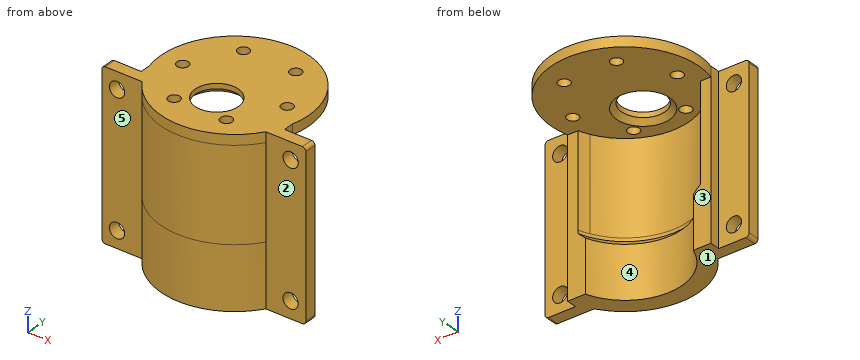
from build123d import *
from build123d.topology import SkipClean

# Parameters (mm, degrees)
BOSS_EXTRUDE1_START     = 94
SKETCH1_R               = 21.9
SKETCH1_R_2             = 1.7
SKETCH1_R_3             = 6.4
BOSS_EXTRUDE1_DEPTH     = 3
BOSS_EXTRUDE2_START     = 91
BOSS_EXTRUDE2_DEPTH     = 27.5
BOSS_EXTRUDE3_START     = 45
BOSS_EXTRUDE3_DEPTH     = 18.5
BOSS_EXTRUDE7_START     = 94
BOSS_EXTRUDE7_DEPTH     = 49
CUT_EXTRUDE5_DEPTH      = 104.301419283
CUT_EXTRUDE5_DEPTH_BACK = 104.301419283
SKETCH4_R               = 2.25
CHAMFER3_SIZE           = 3
CHAMFER4_SIZE           = 1.5
FILLET2_R               = 1


with BuildPart() as part:
    # Sketch1 → Boss-Extrude1 (new body)
    with BuildSketch(Plane.XY.offset(BOSS_EXTRUDE1_START)):
        Circle(SKETCH1_R)
        with Locations((15.475, 0)):
            Circle(SKETCH1_R_2, mode=Mode.SUBTRACT)
        with Locations((7.7375, -13.401743124)):
            Circle(SKETCH1_R_2, mode=Mode.SUBTRACT)
        with Locations((-7.7375, -13.401743124)):
            Circle(SKETCH1_R_2, mode=Mode.SUBTRACT)
        with Locations((-15.475, 0)):
            Circle(SKETCH1_R_2, mode=Mode.SUBTRACT)
        with Locations((-7.7375, 13.401743124)):
            Circle(SKETCH1_R_2, mode=Mode.SUBTRACT)
        with Locations((7.7375, 13.401743124)):
            Circle(SKETCH1_R_2, mode=Mode.SUBTRACT)
        with Locations((0, -7)):
            Circle(SKETCH1_R_3, mode=Mode.SUBTRACT)
    extrude(amount=-BOSS_EXTRUDE1_DEPTH)

    # Sketch1<5> → Boss-Extrude2 (add)
    with BuildSketch(Plane.XY.offset(BOSS_EXTRUDE2_START)):
        with BuildLine():
            ThreePointArc((18.319661569, -12), (19.330787418, -10.292262036), (20.183161298, -8.5))
            Line((20.183161298, -8.5), (16.880758277, -8.5))
            ThreePointArc((16.880758277, -8.5), (0, -18.9), (-16.880758277, -8.5))
            Line((-16.880758277, -8.5), (-20.183161298, -8.5))
            ThreePointArc((-20.183161298, -8.5), (-19.330787418, -10.292262036), (-18.319661569, -12))
            ThreePointArc((-18.319661569, -12), (0, -21.9), (18.319661569, -12))
        make_face()
        with BuildLine():
            Line((-20.183161298, -8.5), (-16.880758277, -8.5))
            ThreePointArc((-16.880758277, -8.5), (-17.545632887, -7.025721786), (-18.082035284, -5.5))
            Line((-18.082035284, -5.5), (-21.198113124, -5.5))
            ThreePointArc((-21.198113124, -5.5), (-20.744938375, -7.018371022), (-20.183161298, -8.5))
        make_face()
        with BuildLine():
            Line((16.880758277, -8.5), (20.183161298, -8.5))
            ThreePointArc((20.183161298, -8.5), (20.744938375, -7.018371022), (21.198113124, -5.5))
            Line((21.198113124, -5.5), (18.082035284, -5.5))
            ThreePointArc((18.082035284, -5.5), (17.545632887, -7.025721786), (16.880758277, -8.5))
        make_face()
    extrude(amount=-BOSS_EXTRUDE2_DEPTH)

    # Sketch1<6> → Boss-Extrude3 (add)
    with SkipClean():  # the faces are left unmerged after this step: merging them gives an invalid solid
        with BuildSketch(Plane.XY.offset(BOSS_EXTRUDE3_START)):
            with BuildLine():
                Line((21.198113124, -5.5), (15.979987484, -5.5))
                ThreePointArc((15.979987484, -5.5), (0, -16.9), (-15.979987484, -5.5))
                Line((-15.979987484, -5.5), (-21.198113124, -5.5))
                ThreePointArc((-21.198113124, -5.5), (0, -21.9), (21.198113124, -5.5))
            make_face()
        extrude(amount=BOSS_EXTRUDE3_DEPTH)

    # Sketch1<11> → Boss-Extrude7 (add)
    with SkipClean():  # the faces are left unmerged after this step: merging them gives an invalid solid
        with BuildSketch(Plane.XY.offset(BOSS_EXTRUDE7_START)):
            with BuildLine():
                ThreePointArc((21.198113124, -5.5), (20.024388359, -8.867574124), (18.319661569, -12))
                Line((18.319661569, -12), (30.183161298, -12))
                Line((30.183161298, -12), (30.183161298, -8.5))
                Line((30.183161298, -8.5), (21.198113124, -8.5))
                Line((21.198113124, -8.5), (21.198113124, -5.5))
            make_face()
            with BuildLine():
                Line((-30.183161298, -12), (-18.319661569, -12))
                ThreePointArc((-18.319661569, -12), (-20.024388359, -8.867574124), (-21.198113124, -5.5))
                Line((-21.198113124, -5.5), (-21.198113124, -8.5))
                Line((-21.198113124, -8.5), (-30.183161298, -8.5))
                Line((-30.183161298, -8.5), (-30.183161298, -12))
            make_face()
        extrude(amount=-BOSS_EXTRUDE7_DEPTH)

    # Sketch4 → Cut-Extrude5 (cut, two sides: drawn at the far end of the back side and taken through both)
    with SkipClean():  # the faces are left unmerged after this step: merging them gives an invalid solid
        with BuildSketch(Plane(origin=(0, -8.5, 0), x_dir=(1, 0, 0), z_dir=(0, 1, 0)).offset(-CUT_EXTRUDE5_DEPTH_BACK)):
            with Locations(Location((-25.690637211, -50, 0), (0, 0, 270))):
                Circle(SKETCH4_R)
            with Locations(Location((-25.690637211, -89, 0), (0, 0, 270))):
                Circle(SKETCH4_R)
            with Locations(Location((25.690637211, -50, 0), (0, 0, 270))):
                Circle(SKETCH4_R)
            with Locations(Location((25.690637211, -89, 0), (0, 0, 270))):
                Circle(SKETCH4_R)
        extrude(amount=CUT_EXTRUDE5_DEPTH + CUT_EXTRUDE5_DEPTH_BACK, mode=Mode.SUBTRACT)

    # Chamfer3
    # the kernel refuses this chamfer: 3 mm, written as the material it takes off along each edge
    with BuildSketch(Plane(origin=(0, 0, 63.5), x_dir=(0.9921367643584464, 0.1251584627915844, 0), z_dir=(-0.1251584627915844, 0.9921367643584464, 0))) as chamfer3_piece_1_section:
        Polygon((16.9 + CHAMFER3_SIZE, 0), (16.9, CHAMFER3_SIZE), (16.9, 0), align=None)
    chamfer3_piece_1 = revolve(axis=Axis((0, 0, 63.5), (0, 0, -1)), revolution_arc=194.379813793, mode=Mode.PRIVATE)
    chamfer3_piece_1 = chamfer3_piece_1 & Plane(origin=(0, 0, 61.502732277), x_dir=(0.8931618135876879, -0.4497354497354555, 0), z_dir=(0, 0, 1)) * Cylinder(18.9, 80, mode=Mode.PRIVATE)
    add(chamfer3_piece_1, mode=Mode.SUBTRACT)

    # Chamfer4
    chamfer4_edges = [part.edges().sort_by_distance(p)[0] for p in [
        (-6.4, -7, 91),
    ]]
    chamfer(chamfer4_edges, length=CHAMFER4_SIZE)

    # Fillet2
    fillet2_edges = [part.edges().sort_by_distance(p)[0] for p in [
        (-30.183161298, -10.25, 45),
        (-30.183161298, -10.25, 94),
        (30.183161298, -10.25, 45),
        (30.183161298, -10.25, 94),
    ]]
    fillet(fillet2_edges, radius=FILLET2_R)


solid = part.part
Build history of the part. All positions in model axes, mm. Face numbers are marked on the shaded views. A direction names the side the tool comes from. Round coordinates to 2 decimals unless told otherwise and drop trailing zeros. Write each loop counter-clockwise with the first axis right and the second up, starting at its lowest first coordinate (ties: lowest second). Pieces come first, ordered by that corner, then holes. Notation, with made-up numbers: (-7.5, -25.75) -> (16.5, -25.75) arc R12 ccw to (16.5, -15.75) -> close; hole circle Ø1 at (-23, -16.75). An arc over 180 degrees is marked (long way). Use one line per item in the form item = value.
Q1. Drop flat-ended pins along their axis: P1, Ø5, axis at x = 20, z = 56.5, coming from the -Y side; P2, Ø3.5, axis at x = 25.69, z = 89, coming from the +Y side; P3, Ø12, axis at x = 0.5, y = 2, coming from the -Z side; P4, Ø3.5, axis at y = -6.5, z = 68.5, coming from the -X side. Give the stop position or say it passes through.
Conclusion:
P1 = -13.17
P2 = through
P3 = 91
P4 = -21.2
Q2. Two-plate mould, pull along X, no slides. Class the marked faces 4 and 5: released by +X, released by -X, zero draft, split by the parting line, or undercut.
Conclusion:
face_4 = undercut
face_5 = zero draft
Q3. Band-saw the part on A-A, the plane z = 89. Write the cut outline in (x, y), then the cut area to 3 significant figures.
Conclusion:
outline = (-30.18, -12) -> (-27.94, -12) -> (-27.94, -8.5) -> (-30.18, -8.5) -> close; (-23.44, -12) -> (-18.32, -12) arc R21.9 ccw to (18.32, -12) -> (23.44, -12) -> (23.44, -8.5) -> (21.2, -8.5) -> (21.2, -5.5) -> (18.08, -5.5) arc R18.9 cw to (-18.08, -5.5) -> (-21.2, -5.5) -> (-21.2, -8.5) -> (-23.44, -8.5) -> close; (27.94, -12) -> (30.18, -12) -> (30.18, -8.5) -> (27.94, -8.5) -> close
area = 206 mm²
Q4. Tool access for the marked faces 1, 2 and 3: list every direction of +Z, -Z, +X, -X, +Y, -Y with a clear straight run to the whole face (end or side of a thin tool).
Conclusion:
face_1 = -Z, +X, -X, +Y, -Y
face_2 = +Z, -Z, +X, -Y
face_3 = -Z, +X, -X, +Y
Q5. Band-saw the part on C-C, the plane z = 66. Write the cut outline in (x, y).
Conclusion:
outline = (-30.18, -12) -> (-18.32, -12) arc R21.9 ccw to (18.32, -12) -> (30.18, -12) -> (30.18, -8.5) -> (21.2, -8.5) -> (21.2, -5.5) -> (18.08, -5.5) arc R18.9 cw to (-18.08, -5.5) -> (-21.2, -5.5) -> (-21.2, -8.5) -> (-30.18, -8.5) -> close
Q6. Band-saw the part on D-D, the plane z = 50. Write the cut outline in (x, y).
Conclusion:
outline = (-30.18, -12) -> (-27.94, -12) -> (-27.94, -8.5) -> (-30.18, -8.5) -> close; (-23.44, -12) -> (-18.32, -12) arc R21.9 ccw to (18.32, -12) -> (23.44, -12) -> (23.44, -8.5) -> (21.2, -8.5) -> (21.2, -5.5) -> (15.98, -5.5) arc R16.9 cw to (-15.98, -5.5) -> (-21.2, -5.5) -> (-21.2, -8.5) -> (-23.44, -8.5) -> close; (27.94, -12) -> (30.18, -12) -> (30.18, -8.5) -> (27.94, -8.5) -> close
Q7. Band-saw the part on B-B, the plane x = 0. Write the cut outline in (y, z), then the cut area to 3 significant figures.
Conclusion:
outline = (-21.9, 45) -> (-16.9, 45) -> (-16.9, 60.5) -> (-18.9, 62.5) -> (-18.9, 91) -> (-14.9, 91) -> (-13.4, 92.5) -> (-13.4, 94) -> (-21.9, 94) -> close; (-0.6, 92.5) -> (0.9, 91) -> (21.9, 91) -> (21.9, 94) -> (-0.6, 94) -> close
area = 262 mm²
Q8. Drill centre lines: L1, parallel to Y at x = 0, z = 93; L2, parallel to Z at x = -12, y = 4.5; L3, parallel to X at y = -10, z = 51. Where is each one in solid material? Low to high.
Conclusion:
L1 = -21.9 to -13.4, -0.6 to 21.9
L2 = 91 to 94
L3 = -30.18 to -27.71, -23.68 to -13.62, 13.62 to 23.68, 27.71 to 30.18
